For this review, take the finished solid that the model builds, in its own axes (mm). A direction names the side the tool comes from. Coordinates: 2 decimals unless noted, no trailing zeros. Loops run counter-clockwise (first coordinate to the right, second up) from the corner with the lowest first, then second, coordinate; pieces in that order, holes last. Notation, with made-up numbers: (89, 29) -> (94, 29) arc R16 ccw to (94, 43) -> close; hole circle Ø1 at (-5, -2). An arc over 180 degrees is marked (long way). Use a Markdown table: item, result.
from build123d import *

# Parameters (mm, degrees)
SKETCH1_R           = 30
BOSS_EXTRUDE1_DEPTH = 10
SKETCH2_W           = 45
SKETCH2_H           = 50
BOSS_EXTRUDE2_DEPTH = 50
SKETCH3_R           = 7.5
BOSS_EXTRUDE3_DEPTH = 30
SKETCH4_R           = 7.5
BOSS_EXTRUDE4_DEPTH = 30
SKETCH5_R           = 7.5
BOSS_EXTRUDE5_DEPTH = 30


with BuildPart() as part:
    # Sketch1 → Boss-Extrude1 (new body)
    with BuildSketch(Plane(origin=(0, 0, 0), x_dir=(1, 0, 0), z_dir=(0, 1, 0))):
        Polygon((-152.5, -62.065153938), (-130, -101.036297108), (130, -101.036297108), (152.5, -62.065153938), (22.5, 163.101451046), (-22.5, 163.101451046), align=None)
        Circle(SKETCH1_R, mode=Mode.SUBTRACT)
    extrude(amount=BOSS_EXTRUDE1_DEPTH)

    # Sketch2 → Boss-Extrude2 (add)
    with BuildSketch(Plane(origin=(0, 10, 0), x_dir=(1, 0, 0), z_dir=(0, 1, 0))):
        with Locations((0, 138.101451046)):
            Rectangle(SKETCH2_W, SKETCH2_H)
        Polygon((-86.698729811, -76.036297108), (-130, -101.036297108), (-152.5, -62.065153938), (-109.198729811, -37.065153938), align=None)
        Polygon((86.698729811, -76.036297108), (130, -101.036297108), (152.5, -62.065153938), (109.198729811, -37.065153938), align=None)
    extrude(amount=BOSS_EXTRUDE2_DEPTH)

    # Sketch3 → Boss-Extrude3 (add)
    with BuildSketch(Plane(origin=(-22.5, 0, -140.601451046), x_dir=(0, 0, -1), z_dir=(1, 0, 0))):
        with Locations((-2.5, 35)):
            Circle(SKETCH3_R)
    extrude(amount=-BOSS_EXTRUDE3_DEPTH)

    # Sketch4 → Boss-Extrude4 (add)
    with BuildSketch(Plane(origin=(133.014428415, 0, 50.815153938), x_dir=(0.866025404, 0, 0.5), z_dir=(-0.5, 0, 0.866025404))):
        with Locations((-2.5, 35)):
            Circle(SKETCH4_R)
    extrude(amount=-BOSS_EXTRUDE4_DEPTH)

    # Sketch5 → Boss-Extrude5 (add)
    with BuildSketch(Plane(origin=(-110.514428415, 0, 89.786297108), x_dir=(-0.866025404, 0, 0.5), z_dir=(-0.5, 0, -0.866025404))):
        with Locations((-2.5, 35)):
            Circle(SKETCH5_R)
    extrude(amount=-BOSS_EXTRUDE5_DEPTH)


solid = part.part
(1) Take a section at C-C on z = 0. Write out the cut boundary in (x, y).
Found:
| item | result |
|---|---|
| outline | (-116.67, 0) -> (-30, 0) -> (-30, 10) -> (-116.67, 10) -> close; (30, 0) -> (116.67, 0) -> (116.67, 10) -> (30, 10) -> close |
(2) For line 1 along Z through (x, y) = (0, 2); line 2 along Y through (x, z) = (109.5, -11.5); line 3 along X through (y, z) = (25, -140.5), list the stretches that pass through material, from the lowest coordinate up.
Found:
| item | result |
|---|---|
| line 1 | z = -163.1 to -30, 30 to 101.04 |
| line 2 | y = 0 to 10 |
| line 3 | x = -22.5 to 22.5 |
(3) Mouldability with a two-part tool opening along Y and no side actions: class faces 4 (the face through (-103.235, 29.094, 85.584)), 5 (the face through (141.092, 29.58, 81.824)), 6 (the face through (-36, 0, -4)) as pulls with the +Y half, pulls with the -Y half, needs draft (parallel to the pull), parting line crosses it, or undercut.
Found:
| item | result |
|---|---|
| face 4 | undercut |
| face 5 | needs draft |
| face 6 | pulls with the -Y half |
(4) Take a section at A-A on x = 0. Write out the cut boundary in (y, z).
Found:
| item | result |
|---|---|
| outline | (0, -163.1) -> (60, -163.1) -> (60, -113.1) -> (10, -113.1) -> (10, -30) -> (0, -30) -> close; (0, 30) -> (10, 30) -> (10, 101.04) -> (0, 101.04) -> close |
(5) For pin 1 Ø15 at (y, z) = (29, -136.5) entering from -X; pin 2 Ø1 at (y, z) = (38.5, 20) entering from -X; pin 3 Ø12 at (x, y) = (-84, 38.5) entering from +Z, all flat-tipped, find the tip position at first contact; note any pin that passes through.
Found:
| item | result |
|---|---|
| pin 1 | stops at x = -52.5 |
| pin 2 | stops at x = 139.85 |
| pin 3 | stops at z = 112.58 |
(6) Take a section at B-B on y = 22. Write out the cut boundary in (x, z), plus the area to 3 significant figures.
Found:
| item | result |
|---|---|
| outline | (-152.5, 62.07) -> (-109.2, 37.07) -> (-86.7, 76.04) -> (-130, 101.04) -> close; (-22.5, -163.1) -> (22.5, -163.1) -> (22.5, -113.1) -> (-22.5, -113.1) -> close; (86.7, 76.04) -> (109.2, 37.07) -> (152.5, 62.07) -> (130, 101.04) -> close |
| area | 6,750 mm^2 |
(7) For faces 1 (the face through (-37.29, 32.13, -145.03)), 2 (the face through (108.046, 34.65, 88.361)), 3 (the face through (98.106, 34.65, 56.278)), list the 3-axis set-ups (+Z, -Z, +X, -X, +Y, -Y) from which the entire face can be reached by the end or side of a thin tool; tool diameter is ignored.
Found:
| item | result |
|---|---|
| face 1 | -X |
| face 2 | +Z, +Y |
| face 3 | -Z, +Y |
(8) Take a section at D-D on y = 39. Write out the cut boundary in (x, z).
Found:
| item | result |
|---|---|
| outline | (-152.5, 62.07) -> (-109.2, 37.07) -> (-86.7, 76.04) -> (-102.86, 85.36) -> (-87.86, 111.34) -> (-98.84, 117.69) -> (-113.84, 91.71) -> (-130, 101.04) -> close; (-52.5, -144.45) -> (-22.5, -144.45) -> (-22.5, -163.1) -> (22.5, -163.1) -> (22.5, -113.1) -> (-22.5, -113.1) -> (-22.5, -131.76) -> (-52.5, -131.76) -> close; (86.7, 76.04) -> (109.2, 37.07) -> (125.36, 46.39) -> (140.36, 20.41) -> (151.34, 26.76) -> (136.34, 52.74) -> (152.5, 62.07) -> (130, 101.04) -> close |
